Verification items for the finished model (mm, model axes). Face numbers are marked on the shaded views. A direction names the side the tool comes from. Give positions to 0.01 mm unless a question says otherwise; leave off trailing zeros. Write each loop counter-clockwise with the first axis right and the second up, starting at its lowest first coordinate (ties: lowest second). Pieces come first, ordered by that corner, then holes. Notation, with made-up numbers: M -9.75,27.25 L 16.25,27.25 A17 cw 16.25,43.25 Z; hole C -4,-23 d3. An arc over 180 degrees is marked long. Write item = value, one per line.
from build123d import *

# Parameters (mm, degrees)
F0_R     = 1.5
F1_DEPTH = 8
F2_R     = 2.75
F3_DEPTH = 3
F5_DEPTH = 1.3
F6_SIZE  = 0.25


with BuildPart() as f1:
    # F0 (on Top) → F1 (new body)
    with BuildSketch(Plane.XY):
        Circle(F0_R)
    extrude(amount=F1_DEPTH)

    # F2 (on Top) → F3 (join)
    with BuildSketch(Plane.XY):
        Circle(F2_R)
    extrude(amount=-F3_DEPTH)

    # F4 (on face) → F5 (cut)
    with BuildSketch(Plane(origin=(0, 0, -3), x_dir=(1, 0, 0), z_dir=(0, 0, -1))):
        Polygon((0.019386, -1.443245), (1.25958, -0.704834), (1.240194, 0.738412), (-0.019386, 1.443245), (-1.25958, 0.704834), (-1.240194, -0.738412), align=None)
    extrude(amount=-F5_DEPTH, mode=Mode.SUBTRACT)

    # F6
    f6_edges = [f1.edges().sort_by_distance(p)[0] for p in [
        (-2.75, 0, -3),
        (-2.75, 0, 0),
        (-1.5, 0, 8),
    ]]
    chamfer(f6_edges, length=F6_SIZE)


solid = f1.part
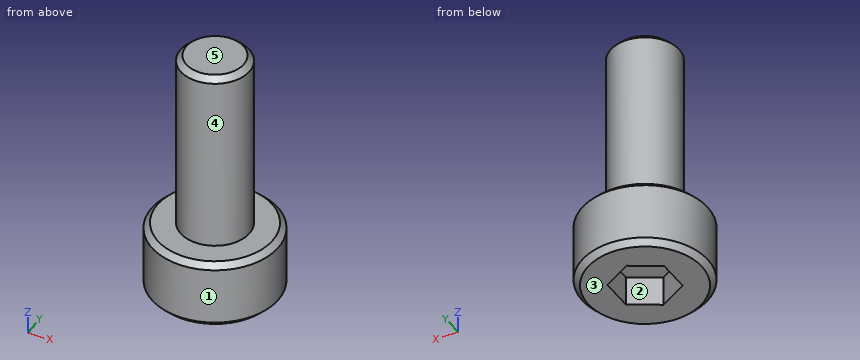
1) Draft check along X on the marked faces 1, 2 and 3. Enter one of: +X half, -X half, draft (parallel to the pull), parting line (faces both ways), or undercut.
From the geometry:
face_1 = parting line
face_2 = undercut
face_3 = draft
2) Cross-section at C-C on z = -0.5. Record the boundary of the cut face in (x, y).
From the geometry:
outline = C 0,0 d5.5
3) Tool access check on the marked faces 4 and 5. Record the directions out of +Z, -Z, +X, -X, +Y, -Y that give a thin tool (end or side, any length) a straight path to the whole face; none if there is none.
From the geometry:
face_4 = +Z
face_5 = +Z, +X, -X, +Y, -Y
4) Cross-section at A-A on z = -2. Record the boundary of the cut face in (x, y), plus the area to 3 significant figures.
From the geometry:
outline = C 0,0 d5.5; hole M -1.26,-0.7 L -0.02,-1.44 L 1.24,-0.74 L 1.26,0.7 L 0.02,1.44 L -1.24,0.74 Z
area = 18.3 mm^2
5) Cross-section at D-D on z = 6.5. Record the boundary of the cut face in (x, y).
From the geometry:
outline = C 0,0 d3
6) Material ranges on probe 1 along Z at (x, y) = (2, 0.2); probe 2 along X at (y, z) = (-0.45, -1.75); probe 3 along Y at (x, z) = (-0.05, 1.5), recorded low to high. Write a range as from..to.
From the geometry:
probe_1 = -3..0
probe_2 = -2.71..-1.26, 1.24..2.71
probe_3 = -1.5..1.5
7) Depth check by flat-ended pin: P1, Ø3, axis at x = 1, z = 6, coming from the -Y side; P2, Ø2, axis at y = 0, z = 6, coming from the -X side; P3, Ø0.8, axis at x = 0, y = -0.5, coming from the -Z side. Enter the tip coordinate at first touch or a pass-through.
From the geometry:
P1 = -1.5
P2 = -1.5
P3 = -1.7
8) Cross-section at B-B on y = 0. Record the boundary of the cut face in (x, z), plus the area to 3 significant figures.
From the geometry:
outline = M -2.75,-2.75 L -2.5,-3 L -1.25,-3 L -1.25,-1.7 L 1.25,-1.7 L 1.25,-3 L 2.5,-3 L 2.75,-2.75 L 2.75,-0.25 L 2.5,0 L 1.5,0 L 1.5,7.75 L 1.25,8 L -1.25,8 L -1.5,7.75 L -1.5,0 L -2.5,0 L -2.75,-0.25 Z
area = 37.1 mm^2
